Check sheet for the modelled part. Datum: model origin and axes. Units: mm. Face numbers are marked on the shaded views. Round coordinates to 2 decimals unless told otherwise and drop trailing zeros. Order: outer loops, then holes, each group sorted by start corner. A loop starts at its lowest first (then second) coordinate and runs counter-clockwise, first axis right, second up. Notation, with made-up numbers: (-8, 41) -> (51, 41) arc R17 ccw to (51, 62) -> close; hole circle Ø2 at (31.25, 21.5). An arc over 180 degrees is marked (long way). Answer in a Markdown table with one row per item. Add a question column.
1. Sectioned sample at B-B, the plane y = 63. Record the boundary of the cut face in (x, z).
2. Depth check by flat-ended pin: P1, Ø3, axis at x = 92, y = 65, coming from the +Z side; P2, Ø3, axis at y = 78.5, z = -28, coming from the +X side; P3, Ø10, axis at x = 64, y = 19, coming from the -Z side; P4, Ø6, axis at y = 22.65, z = -44.16, coming from the +X side. Enter the tip coordinate at first touch or a pass-through.
3. Sectioned sample at A-A, the plane z = -42. Count the separate pieces of the cut face and the enclosed holes in it, then the cut area to 3 significant figures.
4. Material ranges on L1, parallel to X at y = 54, z = -46.5; L2, parallel to Z at x = 72, y = 10; L3, parallel to X at y = 60.5, z = -43, recorded low to high. Write a range as from..to.
5. Draft check along X on the marked faces 1, 2 and 3. Enter one of: +X half, -X half, draft (parallel to the pull), parting line (faces both ways), or undercut.
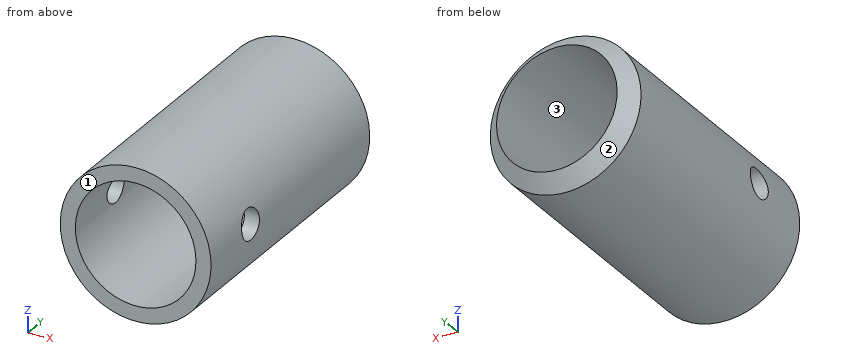
```python
from build123d import *

# Parameters (mm, degrees)
SKETCH2_R           = 25
BOSS_EXTRUDE2_DEPTH = 100
SKETCH3_R           = 20
CUT_EXTRUDE1_DEPTH  = 158.111733872
CHAMFER2_SIZE       = 10
SKETCH4_R           = 5
CUT_EXTRUDE3_DEPTH  = 154.977585945


with BuildPart() as part:
    # Sketch2 → Boss-Extrude2 (new body)
    with BuildSketch(Plane(origin=(0, 0, 0), x_dir=(1, 0, 0), z_dir=(0, 1, 0))):
        with Locations(Location((72.581654817, 46.846486091, 0), (0, 0, 270))):
            Circle(SKETCH2_R)
    extrude(amount=BOSS_EXTRUDE2_DEPTH)

    # Sketch3 → Cut-Extrude1 (cut, through all)
    with BuildSketch(Plane(origin=(0, 100, 0), x_dir=(1, 0, 0), z_dir=(0, 1, 0))):
        with Locations(Location((72.581654817, 46.846486091, 0), (0, 0, 270))):
            Circle(SKETCH3_R)
    extrude(amount=-CUT_EXTRUDE1_DEPTH, mode=Mode.SUBTRACT)

    # Chamfer2
    # the kernel refuses this chamfer: 10 mm, written as the material it takes off along each edge
    with BuildSketch(Plane(origin=(72.581654817, 100, -46.846486091), x_dir=(0, 0, 1), z_dir=(-1, 0, 0))) as chamfer2_piece_1:
        Polygon((25, -CHAMFER2_SIZE), (25 - CHAMFER2_SIZE, 0), (25, 0), align=None)
    revolve(axis=Axis((72.581654817, 100, -46.846486091), (0, 1, 0)), mode=Mode.SUBTRACT)

    # Sketch4 → Cut-Extrude3 (cut, through all)
    with BuildSketch(Plane(origin=(0, 0, 0), x_dir=(0, 0, -1), z_dir=(1, 0, 0))):
        with Locations(Location((44.161502289, 22.651407336, 0), (0, 0, 180))):
            Circle(SKETCH4_R)
    extrude(amount=CUT_EXTRUDE3_DEPTH, mode=Mode.SUBTRACT)


solid = part.part
```
Answer key:
| question | item | result |
|---|---|---|
| 1 | outline | circle Ø50 at (72.58, -46.85); hole circle Ø40 at (72.58, -46.85) |
| 2 | P1 | stops at z = -29.41 |
| 2 | P2 | stops at x = 90.58 |
| 2 | P3 | stops at z = -71.59 |
| 2 | P4 | passes through |
| 3 | separate pieces | 4 |
| 3 | enclosed holes | 0 |
| 3 | area | 855 mm² |
| 4 | L1 | x = 47.58..52.58, 92.58..97.58 |
| 4 | L2 | z = -71.84..-66.84, -26.85..-21.85 |
| 4 | L3 | x = 47.88..52.96, 92.21..97.28 |
| 5 | face 1 | draft |
| 5 | face 2 | parting line |
| 5 | face 3 | undercut |
